Could you check a few things on this model? Use its own coordinates, in mm. Face numbers are marked on the shaded views. A direction names the side the tool comes from. Round coordinates to 2 decimals unless told otherwise and drop trailing zeros. Loops run counter-clockwise (first coordinate to the right, second up) from the corner with the lowest first, then second, coordinate; pieces in that order, holes last. Notation, with made-up numbers: M 27.25,-27 L 55.25,-27 A30 cw 55.25,10 Z; hole C 70,29.25 d4. An arc over 180 degrees is marked long. One line per item, written item: value. Start each with the question number.
Q1. Which directions (+Z, -Z, +X, -X, +Y, -Y) give clear straight access to the entire face, cutting with the end or side of a thin tool? Please do the marked faces 4, 5, 6, 7 and 8.
Q2. Imagine slicing it at B-B (x = -17.5). Please give me the cut outline in (y, z).
Q3. Please list where these lines run through material, in increasing order: line 1 along X through (y, z) = (-3.5, -9); line 2 along X through (y, z) = (3.5, 9); line 3 along Z through (x, y) = (-21, -2).
Q4. Imagine slicing it at D-D (z = -8.25). Give the number of separate pieces and of enclosed holes in the cut face, then the cut area to 3 significant figures.
Q5. Imagine slicing it at C-C (y = -20.5). Please give me the cut outline in (x, z).
Q6. Thinking about a two-plate mould opening in Z: for the marked faces 1, 2 and 3, which applies, released by +Z, released by -Z, zero draft, split by the parting line, or undercut?
Q7. I'm going to push flat-ended pins straight in: pin 1 Ø12 at (x, z) = (-1.5, -3.5) entering from +Y; pin 2 Ø3.5 at (x, z) = (-2.5, -1.5) entering from +Y; pin 3 Ø1.5 at (y, z) = (-13, -2) entering from -X; pin 4 Ø7.5 at (x, z) = (0, 0) entering from -Y. Where does each tip first touch, or does it pass through?
Q8. Imagine slicing it at A-A (y = 2.5). Please give me the cut outline in (x, z).
from build123d import *

# Parameters (mm, degrees)
SKETCH1_R                               = 1.35
BOSS_EXTRUDE1_DEPTH                     = 15.5
BOSS_EXTRUDE1_2_DEPTH                   = 15.5
SKETCH2_R                               = 1.35
BOSS_EXTRUDE2_DEPTH                     = 10
SKETCH4_R                               = 10
BOSS_EXTRUDE3_DEPTH                     = 15
CBORE_FOR_M5_HEX_HEAD_BOLT1_D           = 5.5
CBORE_FOR_M5_HEX_HEAD_BOLT1_CBORE_D     = 12.24
CBORE_FOR_M5_HEX_HEAD_BOLT1_CBORE_DEPTH = 5
FILLET1_R                               = 3


with BuildPart() as part:
    # Sketch1 → Boss-Extrude1 (new body)
    with BuildSketch(Plane(origin=(0, 0, 0), x_dir=(1, 0, 0), z_dir=(0, 1, 0))):
        with BuildLine():
            Line((21, 12), (16.5, 12))
            Line((16.5, 12), (16.5, -12))
            Line((16.5, -12), (21, -12))
            ThreePointArc((21, -12), (23.121320344, -11.121320344), (24, -9))
            Line((24, -9), (24, 9))
            ThreePointArc((24, 9), (23.121320344, 11.121320344), (21, 12))
        make_face()
        with Locations((21, -9)):
            Circle(SKETCH1_R, mode=Mode.SUBTRACT)
        with Locations((21, 9)):
            Circle(SKETCH1_R, mode=Mode.SUBTRACT)
    extrude(amount=BOSS_EXTRUDE1_DEPTH)



with BuildPart() as body_2:
    # Sketch1 → Boss-Extrude1 2 (new body)
    with BuildSketch(Plane(origin=(0, 0, 0), x_dir=(1, 0, 0), z_dir=(0, 1, 0))):
        with BuildLine():
            Line((-16.5, 12), (-21, 12))
            ThreePointArc((-21, 12), (-23.121320344, 11.121320344), (-24, 9))
            Line((-24, 9), (-24, -9))
            ThreePointArc((-24, -9), (-23.121320344, -11.121320344), (-21, -12))
            Line((-21, -12), (-16.5, -12))
            Line((-16.5, -12), (-16.5, 12))
        make_face()
        with Locations((-21, -9)):
            Circle(SKETCH1_R, mode=Mode.SUBTRACT)
        with Locations((-21, 9)):
            Circle(SKETCH1_R, mode=Mode.SUBTRACT)
    extrude(amount=BOSS_EXTRUDE1_2_DEPTH)


with BuildPart() as part_1:
    add(part.part)

    add(body_2.part)  # Boss-Extrude2 merges body 2
    # Sketch2 → Boss-Extrude2 (add)
    with BuildSketch(Plane(origin=(0, 0, 0), x_dir=(1, 0, 0), z_dir=(0, 1, 0))):
        with BuildLine():
            Line((24, 9), (24, -9))
            ThreePointArc((24, -9), (23.121320344, -11.121320344), (21, -12))
            Line((21, -12), (16.5, -12))
            Line((16.5, -12), (-16.5, -12))
            Line((-16.5, -12), (-21, -12))
            ThreePointArc((-21, -12), (-23.121320344, -11.121320344), (-24, -9))
            Line((-24, -9), (-24, 9))
            ThreePointArc((-24, 9), (-23.121320344, 11.121320344), (-21, 12))
            Line((-21, 12), (-16.5, 12))
            Line((-16.5, 12), (16.5, 12))
            Line((16.5, 12), (21, 12))
            ThreePointArc((21, 12), (23.121320344, 11.121320344), (24, 9))
        make_face()
        with Locations((21, 9)):
            Circle(SKETCH2_R, mode=Mode.SUBTRACT)
        with Locations((21, -9)):
            Circle(SKETCH2_R, mode=Mode.SUBTRACT)
        with Locations((-21, 9)):
            Circle(SKETCH2_R, mode=Mode.SUBTRACT)
        with Locations((-21, -9)):
            Circle(SKETCH2_R, mode=Mode.SUBTRACT)
    extrude(amount=-BOSS_EXTRUDE2_DEPTH)

    # Sketch4 → Boss-Extrude3 (add)
    with BuildSketch(Plane.XZ.offset(10)):
        Circle(SKETCH4_R)
    extrude(amount=BOSS_EXTRUDE3_DEPTH)

    # CBORE for M5 Hex Head Bolt1 (through all)
    with Locations(Plane.ZX):
        with Locations((0, 0)):
            CounterBoreHole(CBORE_FOR_M5_HEX_HEAD_BOLT1_D / 2, CBORE_FOR_M5_HEX_HEAD_BOLT1_CBORE_D / 2, CBORE_FOR_M5_HEX_HEAD_BOLT1_CBORE_DEPTH)

    # Fillet1
    fillet1_edges = [part_1.edges().sort_by_distance(p)[0] for p in [
        (-16.5, 7.75, -12),
        (-16.5, 7.75, 12),
        (16.5, 7.75, -12),
        (16.5, 7.75, 12),
        (-10, -10, 0),
    ]]
    fillet(fillet1_edges, radius=FILLET1_R)


solid = part_1.part
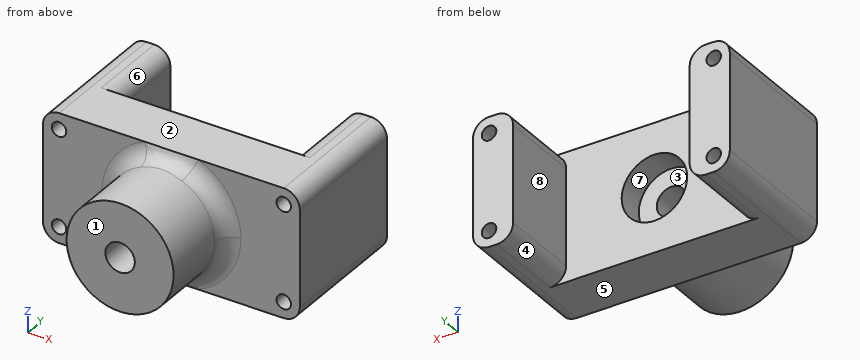
Report:
1. face 4: -Z, +Y
1. face 5: -Z, +X, -X, +Y, -Y
1. face 6: +Z, +Y
1. face 7: +Y
1. face 8: +Z, -Z, +Y
2. outline: M -10,-12 L 0,-12 L 0,-11.24 L 15.5,-11.24 L 15.5,11.24 L 0,11.24 L 0,12 L -10,12 Z
3. line 1: x = -24 to -22.35, -19.65 to 19.65, 22.35 to 24
3. line 2: x = -24 to -22.35, -19.65 to -16.5, 16.5 to 19.65, 22.35 to 24
3. line 3: z = -12 to -10.35, -7.65 to 7.65, 10.35 to 12
4. separate pieces: 3
4. enclosed holes: 0
4. area: 774 mm²
5. outline: C 0,0 d20; hole C 0,0 d5.5
6. face 1: zero draft
6. face 2: released by +Z
6. face 3: undercut
7. pin 1: stops at y = 0
7. pin 2: stops at y = -5
7. pin 3: stops at x = -9.94
7. pin 4: stops at y = -25
8. outline: M -24,-9 A3 ccw -21,-12 L -19.5,-12 A3 ccw -16.5,-9 L -16.5,9 A3 ccw -19.5,12 L -21,12 A3 ccw -24,9 Z; M 16.5,-9 A3 ccw 19.5,-12 L 21,-12 A3 ccw 24,-9 L 24,9 A3 ccw 21,12 L 19.5,12 A3 ccw 16.5,9 Z; hole C -21,-9 d2.7; hole C -21,9 d2.7; hole C 21,-9 d2.7; hole C 21,9 d2.7
